Read the model definition and answer for the solid it produces. Units are mm, in the model's axes. Coordinates: 2 decimals unless noted, no trailing zeros. Loops run counter-clockwise (first coordinate to the right, second up) from the corner with the lowest first, then second, coordinate; pieces in that order, holes last. Notation, with made-up numbers: (77, 21.5) - (90, 21.5) arc R11 ccw to (90, 37.5) - close; hole circle Ø4 at (56.25, 1.5). An arc over 180 degrees is marked (long way). Use one line per item in the form item = value.
Autodesk Inventor part; units mm, degrees
ref_plane "Plano inicial" through (0, 0, 0) normal (0, 0, 1) x (1, 0, 0)
ref_plane "Plano final" through (0, 0, 800) normal (0, 0, 1) x (1, 0, 0)
ref_plane "YZ Plane" through (0, 0, 0) normal (1, 0, 0) x (0, 1, 0)
ref_plane "Plano inicial" through (0, 0, 0) normal (0, 0, 1) x (1, 0, 0)
ref_plane "Plano final" through (0, 0, 800) normal (0, 0, 1) x (1, 0, 0)
sketch "Esboço" plane through (0, 0, 0) normal (0, 0, 1) x (1, 0, 0)
  line L0 (-12.5, -21.25) -> (-12.5, 21.25)
  line L1 (-8.75, 25) -> (8.75, 25)
  line L2 (12.5, 21.25) -> (12.5, -21.25)
  line L3 (8.75, -25) -> (-8.75, -25)
  arc A0 (-12.5, -21.25) -> (-8.75, -25) centre (-8.75, -21.25) ccw
  arc A1 (-8.75, 25) -> (-12.5, 21.25) centre (-8.75, 21.25) ccw
  arc A2 (12.5, 21.25) -> (8.75, 25) centre (8.75, 21.25) ccw
  arc A3 (8.75, -25) -> (12.5, -21.25) centre (8.75, -21.25) ccw
  line L4 (-7.5, 22.5) -> (7.5, 22.5)
  line L5 (10, 20) -> (10, -20)
  line L6 (7.5, -22.5) -> (-7.5, -22.5)
  line L7 (-10, -20) -> (-10, 20)
  line L8 (0, 36.0873) -> (0, -36.0873) construction
  line L9 (-18.5873, 0) -> (18.5873, 0) construction
  arc A4 (-10, -20) -> (-7.5, -22.5) centre (-7.5, -20) ccw
  arc A5 (-7.5, 22.5) -> (-10, 20) centre (-7.5, 20) ccw
  arc A6 (10, 20) -> (7.5, 22.5) centre (7.5, 20) ccw
  arc A7 (7.5, -22.5) -> (10, -20) centre (7.5, -20) ccw
  dimension "d7" = 3.75
  dimension "d10" = 50
  dimension "d11" = 25
  dimension "d12" = 2.5
  dimension "d15" = 25
  dimension "d16" = 12.5
  dimension "d19" = 2.5
  dimension "d20" = 2.5
extrude "Corpo" add sketch "Esboço" along normal up to surface (800 mm away) from surface at 0
sketch "Sketch3" plane through (0, 0, 0) normal (0, 0, 1) x (1, 0, 0)
  line L0 (0, 0) -> (10, 0)
ref_plane "Work Plane3" through (0, 0, 0) normal (0, -1, 0) x (1, 0, 0)
sketch "Sketch4" plane through (0, 0, 0) normal (0, -1, 0) x (1, 0, 0)
  line L0 (-2, 0) -> (12, 0)
  line L1 (-2, 800) -> (12, 800)
  dimension "d18" = 800
equation "\"d7\" = G_IR"
equation "\"d10\" = G_H"
equation "\"d11\" = G_W"
equation "\"d12\" = G_T"
equation "\"d15\" = 0.5 * d10"
equation "\"d16\" = 0.5 * d11"
equation "\"d19\" = G_T"
equation "\"d20\" = G_T"
equation "\"d3\" = G_L"
equation "\"G_W\" = 25"
equation "\"G_H\" = 50"
equation "\"G_T\" = 2.5"
equation "\"G_IR\" = 3.75"
equation "\"G_L\" = d18"
equation "\"G_OFFSET_START\" = 0"
equation "\"G_OFFSET_END\" = 0"
properties part number "EN 10210-2 - 50 x 25 x 2,5 - 800" material "Aço, suave"
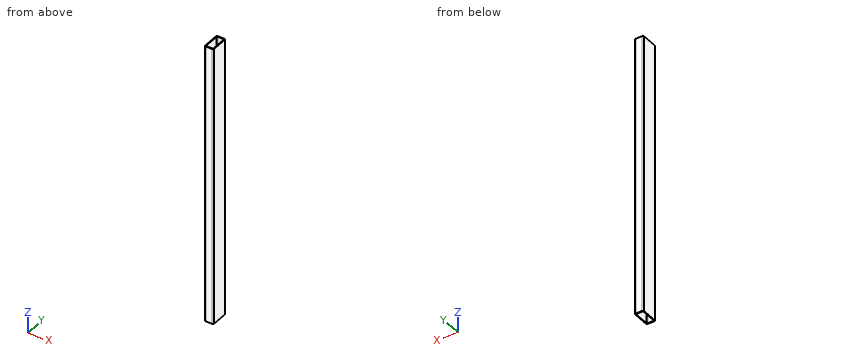
Item 1: The part is cut by section A-A on y = -5. Give the vertices of the cut face in (x, z), plus the area to 3 significant figures.
Results below:
outline = (-12.5, 0) - (-10, 0) - (-10, 800) - (-12.5, 800) - close; (10, 0) - (12.5, 0) - (12.5, 800) - (10, 800) - close
area = 4,000 mm²
Item 2: Find the intervals of material crossed by L1, parallel to X at y = 3.5, z = 564; L2, parallel to Y at x = -0.75, z = 252; L3, parallel to X at y = 21, z = 659.5, in increasing order.
Results below:
L1 = -12.5 to -10, 10 to 12.5
L2 = -25 to -22.5, 22.5 to 25
L3 = -12.5 to -9.79, 9.79 to 12.5
Item 3: The part is cut by section C-C on x = -3.5. Give the vertices of the cut face in (y, z), plus the area to 3 significant figures.
Results below:
outline = (-25, 0) - (-22.5, 0) - (-22.5, 800) - (-25, 800) - close; (22.5, 0) - (25, 0) - (25, 800) - (22.5, 800) - close
area = 4,000 mm²
Item 4: The part is cut by section B-B on z = 591. Give the vertices of the cut face in (x, y).
Results below:
outline = (-12.5, -21.25) arc R3.75 ccw to (-8.75, -25) - (8.75, -25) arc R3.75 ccw to (12.5, -21.25) - (12.5, 21.25) arc R3.75 ccw to (8.75, 25) - (-8.75, 25) arc R3.75 ccw to (-12.5, 21.25) - close; hole (-10, -20) arc R2.5 ccw to (-7.5, -22.5) - (7.5, -22.5) arc R2.5 ccw to (10, -20) - (10, 20) arc R2.5 ccw to (7.5, 22.5) - (-7.5, 22.5) arc R2.5 ccw to (-10, 20) - close
